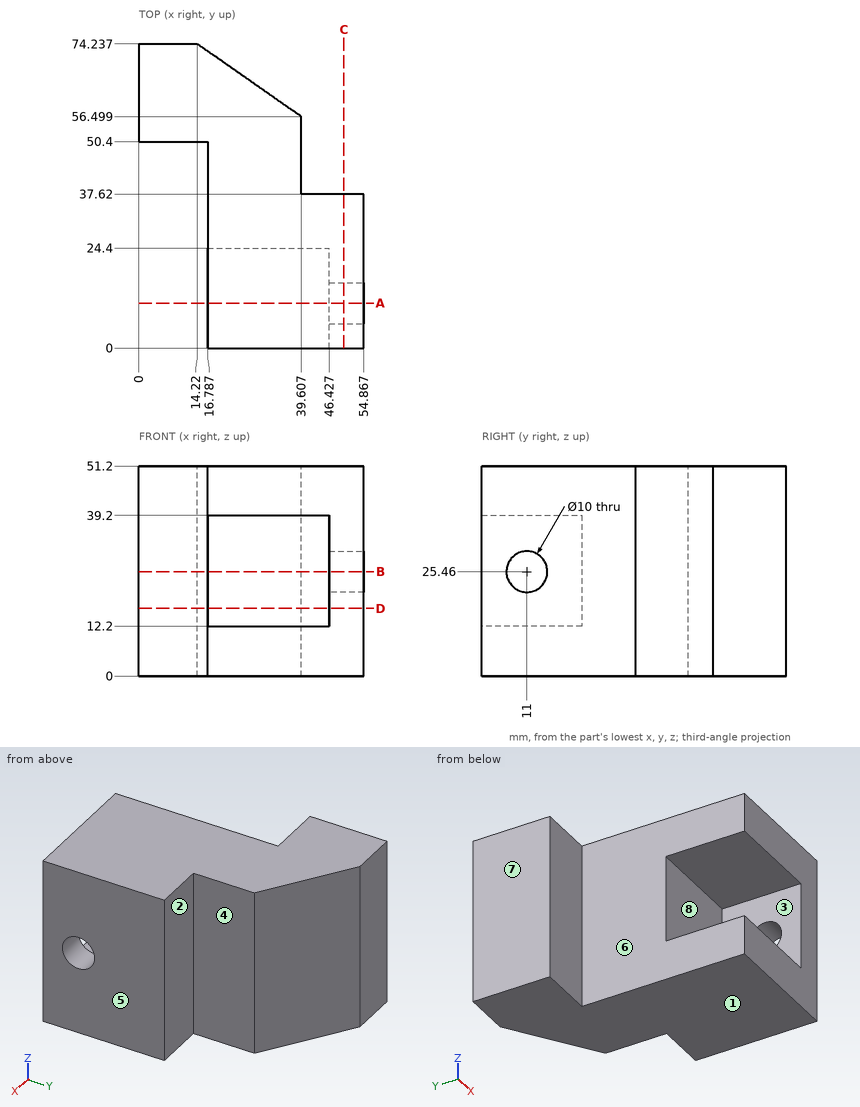
Here's the drawing with two shaded views (mm, measured from the low corner). I have some questions. A direction names the side the tool comes from. Coordinates: 2 decimals unless noted, no trailing zeros. Loops run counter-clockwise (first coordinate to the right, second up) from the corner with the lowest first, then second, coordinate; pieces in that order, holes last. Notation, with made-up numbers: M 6.25,7.25 L 46.25,7.25 A8 ccw 46.25,15.25 Z; hole C 48,4.5 d10. An arc over 180 degrees is marked long. Answer as CSV lines item,"result". Start each with the question number.
1. For pin 1 Ø6 at (y, z) = (37.5, 31) entering from -X; pin 2 Ø4 at (x, z) = (33.5, 27.5) entering from +Y; pin 3 Ø7.5 at (y, z) = (16.5, 30) entering from -X, each with a flat end and sliding along its axis, tell me the tip position at first contact or that it passes through.
2. Suppose I cut it at D-D, the plane z = 16.5. List the corners of the cut face in (x, y) for me, plus the area to 3 significant figures.
3. If I drill on probe 1 along Z at (x, y) = (31.5, 13); probe 2 along Y at (x, z) = (52, 25); probe 3 along X at (y, z) = (52.5, 34), over which ranges is the centre line in solid material (lowest first)? Write a range as [from, to].
4. Thinking about a two-plate mould opening in Z: for the marked faces 1, 2 and 3, which applies, +Z half, -Z half, draft (parallel to the pull), parting line (faces both ways), or undercut?
5. Suppose I cut it at A-A, the plane y = 11. List the corners of the cut face in (x, z) for me, plus the area to 4 significant figures.
6. For the marked faces 4, 5, 6, 7 and 8, which set-ups out of +Z, -Z, +X, -X, +Y, -Y let a thin tool reach every point of the face, with its end or its side?
7. Suppose I cut it at B-B, the plane z = 25.46. List the corners of the cut face in (x, y) for me.
8. Suppose I cut it at C-C, the plane x = 50. List the corners of the cut face in (y, z) for me, plus the area to 3 significant figures.
Output:
1,pin 1,"stops at x = 16.79"
1,pin 2,"stops at y = 62.16"
1,pin 3,"stops at x = 46.43"
2,outline,"M 0,50.4 L 16.79,50.4 L 16.79,24.4 L 46.43,24.4 L 46.43,0 L 54.87,0 L 54.87,37.62 L 39.61,37.62 L 39.61,56.5 L 14.22,74.24 L 0,74.24 Z"
2,area,"1,720 mm^2"
3,probe 1,"z = [0, 12.2], [39.2, 51.2]"
3,probe 2,"y = [0, 6.02], [15.98, 37.62]"
3,probe 3,"x = [0, 39.61]"
4,face 1,"-Z half"
4,face 2,"draft"
4,face 3,"undercut"
5,outline,"M 16.79,0 L 54.87,0 L 54.87,20.46 L 46.43,20.46 L 46.43,12.2 L 16.79,12.2 Z; M 16.79,39.2 L 46.43,39.2 L 46.43,30.46 L 54.87,30.46 L 54.87,51.2 L 16.79,51.2 Z"
5,area,"1,065 mm^2"
6,face 4,"+Z, -Z, +X, +Y"
6,face 5,"+Z, -Z, +X, +Y, -Y"
6,face 6,"+Z, -Z, -X, -Y"
6,face 7,"+Z, -Z, -X, +Y, -Y"
6,face 8,"-X, -Y"
7,outline,"M 0,50.4 L 16.79,50.4 L 16.79,24.4 L 46.43,24.4 L 46.43,16 L 54.87,16 L 54.87,37.62 L 39.61,37.62 L 39.61,56.5 L 14.22,74.24 L 0,74.24 Z; M 46.43,0 L 54.87,0 L 54.87,6 L 46.43,6 Z"
8,outline,"M 0,0 L 37.62,0 L 37.62,51.2 L 0,51.2 Z; hole C 11,25.46 d10"
8,area,"1,850 mm^2"
